Check sheet for the modelled part. Datum: model origin and axes. Units: mm. Coordinates: 2 decimals unless noted, no trailing zeros. Loops run counter-clockwise (first coordinate to the right, second up) from the corner with the lowest first, then second, coordinate; pieces in that order, holes last. Notation, with made-up numbers: M -31.75,-32.75 L -23.75,-32.75 A27 cw -23.75,-16.75 Z; hole C 81,21.5 d11. An arc over 180 degrees is marked long. Return JSON: item names as keys, results as strings.
from build123d import *

# Parameters (mm, degrees)
SKETCH_1_W      = 196
SKETCH_1_H      = 196
SKETCH_1_R      = 5.5
SKETCH_1_R_2    = 5.499997081
SKETCH_1_R_3    = 13
EXTRUDE_1_DEPTH = 17


with BuildPart() as part:
    # Эскиз1 → Бобышка-Вытянуть1 (new body)
    with BuildSketch(Plane.XY.offset(17)):
        Rectangle(SKETCH_1_W, SKETCH_1_H)
        with Locations(Location((-50, -77, 0), (0, 0, 180))):
            Circle(SKETCH_1_R, mode=Mode.SUBTRACT)
        with Locations(Location((-50.000002921, 76.99985459, 0), (0, 0, 180))):
            Circle(SKETCH_1_R_2, mode=Mode.SUBTRACT)
        with Locations(Location((50, -77, 0), (0, 0, 180))):
            Circle(SKETCH_1_R, mode=Mode.SUBTRACT)
        with Locations(Location((49.999997079, 76.99985459, 0), (0, 0, 180))):
            Circle(SKETCH_1_R_2, mode=Mode.SUBTRACT)
        with Locations(Location((-76, 77, 0), (0, 0, 180))):
            Circle(SKETCH_1_R_3, mode=Mode.SUBTRACT)
        with Locations(Location((-76, -77, 0), (0, 0, 180))):
            Circle(SKETCH_1_R_3, mode=Mode.SUBTRACT)
        with Locations(Location((76, -77, 0), (0, 0, 180))):
            Circle(SKETCH_1_R_3, mode=Mode.SUBTRACT)
        with Locations(Location((76, 77, 0), (0, 0, 180))):
            Circle(SKETCH_1_R_3, mode=Mode.SUBTRACT)
    extrude(amount=-EXTRUDE_1_DEPTH)


solid = part.part
1) Section check D-D on x = 50. Record the cut outline in (y, z).
Answers:
{"outline": "M -98,0 L -82.5,0 L -82.5,17 L -98,17 Z; M -71.5,0 L 71.5,0 L 71.5,17 L -71.5,17 Z; M 82.5,0 L 98,0 L 98,17 L 82.5,17 Z"}
2) Section check C-C on z = 13. Count the separate pieces of the cut face and the enclosed holes in it, then the cut area to 3 significant figures.
Answers:
{"separate pieces": "1", "enclosed holes": "8", "area": "35,900 mm²"}
3) Section check B-B on x = -76. Record the cut outline in (y, z).
Answers:
{"outline": "M -98,0 L -90,0 L -90,17 L -98,17 Z; M -64,0 L 64,0 L 64,17 L -64,17 Z; M 90,0 L 98,0 L 98,17 L 90,17 Z"}
4) Section check A-A on y = -77. Record the cut outline in (x, z), then the cut area to 3 significant figures.
Answers:
{"outline": "M -98,0 L -89,0 L -89,17 L -98,17 Z; M -63,0 L -55.5,0 L -55.5,17 L -63,17 Z; M -44.5,0 L 44.5,0 L 44.5,17 L -44.5,17 Z; M 55.5,0 L 63,0 L 63,17 L 55.5,17 Z; M 89,0 L 98,0 L 98,17 L 89,17 Z", "area": "2,070 mm²"}
5) Scan lines: line 1 along X through (y, z) = (-77, 12.5); line 2 along Y through (x, z) = (50, 10.5); line 3 along Y through (x, z) = (76, 8.25). Record each from-to range of solid material in increasing order. Write a range as [from, to].
Answers:
{"line 1": "[-98, -89], [-63, -55.5], [-44.5, 44.5], [55.5, 63], [89, 98]", "line 2": "[-98, -82.5], [-71.5, 71.5], [82.5, 98]", "line 3": "[-98, -90], [-64, 64], [90, 98]"}
